Verification items for this drawing (mm, ordinates from the low corner). A direction names the side the tool comes from. Give positions to 0.01 mm unless a question says otherwise; leave off trailing zeros. Loops run counter-clockwise (first coordinate to the right, second up) from the corner with the lowest first, then second, coordinate; pieces in that order, holes last. Notation, with made-up numbers: (-3, -32) -> (30, -32) arc R10 cw to (30, -22) -> close; hole circle Ø1 at (8.5, 29.25). An arc over 180 degrees is marked (long way). Write each question's results on one line, items separated by ' | '. Start each with the question number.
Item 1: Cross-section at A-A on x = 10. Enter the section's corners in (y, z).
Item 2: Access from +Z, -Z, +X, -X, +Y, -Y to the whole of each face (thin tool, end or side, straight path). Record for the marked faces 4 and 5.
Item 3: Gauge pin test, flat ends, axial feed: pin 1 Ø2 at (x, y) = (11, 9.5) entering from -Z; pin 2 Ø4 at (y, z) = (3, 6) entering from -X; pin 3 Ø6 at (x, z) = (13, 4) entering from +Y. Record the tip position at first contact, or that the pin passes through.
Item 4: Cross-section at C-C on z = 2.5. Enter the section's corners in (x, y), then the cut area to 3 significant figures.
Item 5: Scan lines: line 1 along Y through (x, z) = (10, 3.05); line 2 along Z through (x, y) = (9.5, 12); line 3 along X through (y, z) = (9.5, 4.25). Record each from-to range of solid material in increasing order.
Item 6: Mould release check, pull along Y, two halves, no side actions. Record for the marked faces 1, 2 and 3: pulls with the +Y half, pulls with the -Y half, needs draft (parallel to the pull), parting line crosses it, or undercut.
Item 7: Cross-section at D-D on z = 7.5. Enter the section's corners in (x, y).
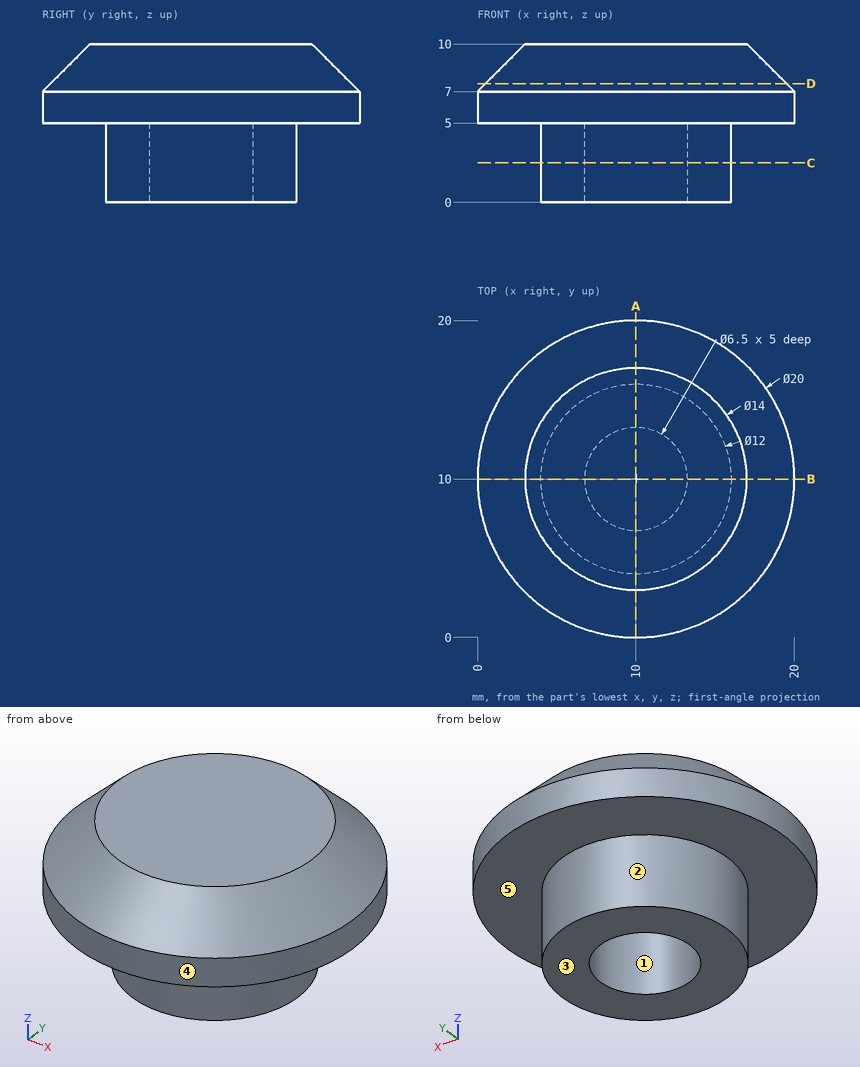
Answer sheet:
1) outline: (0, 5) -> (4, 5) -> (4, 0) -> (6.75, 0) -> (6.75, 5) -> (13.25, 5) -> (13.25, 0) -> (16, 0) -> (16, 5) -> (20, 5) -> (20, 7) -> (17, 10) -> (3, 10) -> (0, 7) -> close
2) face 4: +Z, -Z | face 5: -Z
3) pin 1: stops at z = 5 | pin 2: stops at x = 1.34 | pin 3: stops at y = 20
4) outline: circle Ø12 at (10, 10); hole circle Ø6.5 at (10, 10) | area: 79.9 mm²
5) line 1: y = 4 to 6.75, 13.25 to 16 | line 2: z = 5 to 10 | line 3: x = 4.02 to 6.79, 13.21 to 15.98
6) face 1: undercut | face 2: parting line crosses it | face 3: needs draft
7) outline: circle Ø19 at (10, 10)
